Design review of the part built by this model. Coordinates are the model's own, in mm. Coordinates: 2 decimals unless noted, no trailing zeros. Write each loop counter-clockwise with the first axis right and the second up, starting at its lowest first coordinate (ties: lowest second). Pieces come first, ordered by that corner, then holes. Notation, with made-up numbers: M -17.5,66.5 L 6.5,66.5 A12 cw 6.5,76.5 Z; hole C 57,37 d2. An arc over 180 degrees is marked long. Return JSON: item names as keys, results as strings. Group by question number.
```python
from build123d import *

# Parameters (mm, degrees)
SKETCH2_W           = 240
SKETCH2_H           = 115
SKETCH2_W_2         = 30
SKETCH2_H_2         = 5
BOSS_EXTRUDE1_DEPTH = 5


with BuildPart() as part:
    # Sketch2 → Boss-Extrude1 (new body)
    with BuildSketch(Plane.XY):
        Rectangle(SKETCH2_W, SKETCH2_H)
        with Locations((-94.565217391, 50)):
            Rectangle(SKETCH2_W_2, SKETCH2_H_2, mode=Mode.SUBTRACT)
        with Locations((0.434782609, 50)):
            Rectangle(SKETCH2_W_2, SKETCH2_H_2, mode=Mode.SUBTRACT)
        with Locations((95, 50)):
            Rectangle(SKETCH2_W_2, SKETCH2_H_2, mode=Mode.SUBTRACT)
        with Locations((-95, 10)):
            Rectangle(SKETCH2_W_2, SKETCH2_H_2, mode=Mode.SUBTRACT)
        with Locations((0, 10)):
            Rectangle(SKETCH2_W_2, SKETCH2_H_2, mode=Mode.SUBTRACT)
        with Locations((95, 10)):
            Rectangle(SKETCH2_W_2, SKETCH2_H_2, mode=Mode.SUBTRACT)
        with Locations((-95, -45)):
            Rectangle(SKETCH2_W_2, SKETCH2_H_2, mode=Mode.SUBTRACT)
        with Locations((0, -45)):
            Rectangle(SKETCH2_W_2, SKETCH2_H_2, mode=Mode.SUBTRACT)
        with Locations((95, -45)):
            Rectangle(SKETCH2_W_2, SKETCH2_H_2, mode=Mode.SUBTRACT)
    extrude(amount=BOSS_EXTRUDE1_DEPTH)


solid = part.part
```
Item 1: Add section B-B (z = 1.25). Count the separate pieces of the cut face and the enclosed holes in it, plus the area to 4 significant figures.
Item 2: Add section A-A (x = 8). Write out the cut boundary in (y, z).
Item 3: For line 1 (X direction, y = -47, z = 1.05); line 2 (Y direction, x = -87, z = 1.2); line 3 (X direction, y = 48, z = 4.15), list the stretches that pass through material, from the lowest coordinate up.
Item 4: The part is to be moulded in two halves that separate along X. For faces 1 (the flat face through (-2, 57.5, 2)), 2 (the flat face through (0, 47.5, 2)), say which applies: pulls with the +X half, pulls with the -X half, needs draft (parallel to the pull), parting line crosses it, or undercut.
Geometry check:
{
 "1": {"separate pieces": "1", "enclosed holes": "9", "area": "26,250 mm^2"},
 "2": {"outline": "M -57.5,0 L -47.5,0 L -47.5,5 L -57.5,5 Z; M -42.5,0 L 7.5,0 L 7.5,5 L -42.5,5 Z; M 12.5,0 L 47.5,0 L 47.5,5 L 12.5,5 Z; M 52.5,0 L 57.5,0 L 57.5,5 L 52.5,5 Z"},
 "3": {"line 1": "-120 to -110, -80 to -15, 15 to 80, 110 to 120", "line 2": "-57.5 to -47.5, -42.5 to 7.5, 12.5 to 47.5, 52.5 to 57.5", "line 3": "-120 to -109.57, -79.57 to -14.57, 15.43 to 80, 110 to 120"},
 "4": {"face 1": "needs draft", "face 2": "undercut"}
}
